Work out the finished part from the listing and answer in its coordinate system (mm). Face numbers are marked on the shaded views. Give positions to 0.01 mm unless a question says otherwise; leave off trailing zeros. Loops run counter-clockwise (first coordinate to the right, second up) from the corner with the lowest first, then second, coordinate; pieces in that order, holes last. Notation, with made-up numbers: (-17.75, 20) -> (32.25, 20) arc R24 cw to (32.25, 57) -> close; hole circle Ø9 at (-37, 57.5). An arc over 180 degrees is marked (long way). Answer as CSV lines item,"result". Start each with the question number.
1. Flat-ended cylindrical pins translate along their axes: pin 1 Ø2 at (x, y) = (-6, 1.5) entering from +Z; pin 2 Ø4 at (x, z) = (0, 0) entering from +Y; pin 3 Ø12 at (x, z) = (-5, -23) entering from +Y; pin 4 Ø4 at (x, y) = (-27.5, 5) entering from -Z. Find the tip coordinate at first contact, or state that the pin passes through.
2. Find section C-C, the plane y = 4. Give the vertices of the cut face in (x, z).
3. Find section D-D, the plane x = -6. Give the vertices of the cut face in (y, z), and give its area (3 significant figures).
4. Find the intervals of material crossed by line 1 along X through (y, z) = (6.5, -35); line 2 along Z through (x, y) = (-9.5, 8.75); line 3 along Z through (x, y) = (-14, 5.5), in increasing order.
5. Determine the mould class of the marked faces 1 and 2 for opening direction X: +X half, -X half, draft (parallel to the pull), parting line (faces both ways), or undercut.
6. Find section A-A, the plane x = 0. Give the vertices of the cut face in (y, z).
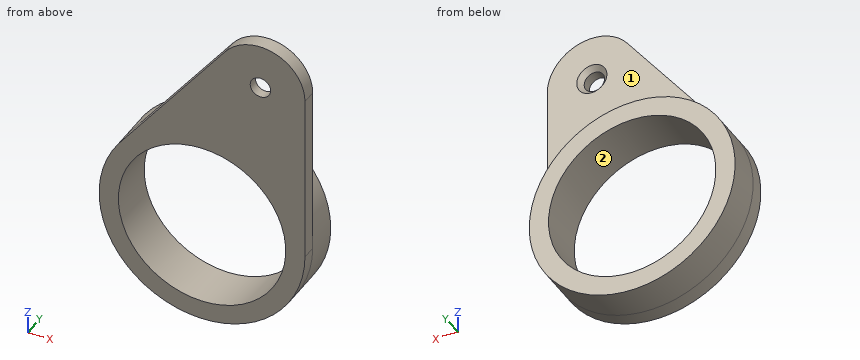
from build123d import *
from build123d.topology import SkipClean

# Parameters (mm, degrees)
SKETCH1_R           = 17.2
SKETCH1_R_2         = 2.1
BOSS_EXTRUDE1_DEPTH = 3
CHAMFER1_SIZE       = 1
SKETCH2_R           = 21.154971589
SKETCH2_R_2         = 17.2
BOSS_EXTRUDE2_DEPTH = 7


with BuildPart() as part:
    # Sketch1 → Boss-Extrude1 (new body)
    with BuildSketch(Plane(origin=(0, 0, 0), x_dir=(1, 0, 0), z_dir=(0, 1, 0))):
        with BuildLine():
            ThreePointArc((-29.22705293, 22.721503746), (-18.44573532, 55.149077376), (9.154971589, 35))
            Line((9.154971589, 35), (9.154971589, 0))
            ThreePointArc((9.154971589, 0), (2.966995431, -8.660856938), (-7.231849971, -5.613719871))
            Line((-7.231849971, -5.613719871), (-29.22705293, 22.721503746))
        make_face()
        with Locations(Location((-12, 35, 0), (0, 0, 270))):
            Circle(SKETCH1_R, mode=Mode.SUBTRACT)
        with Locations(Location((0, 0, 0), (0, 0, 270))):
            Circle(SKETCH1_R_2, mode=Mode.SUBTRACT)
    extrude(amount=BOSS_EXTRUDE1_DEPTH)

    # Chamfer1
    chamfer1_edges = [part.edges().sort_by_distance(p)[0] for p in [
        (0, 3, -2.1),
    ]]
    chamfer(chamfer1_edges, length=CHAMFER1_SIZE)

    # Sketch2 → Boss-Extrude2 (add)
    with SkipClean():  # the faces are left unmerged after this step: merging them gives an invalid solid
        with BuildSketch(Plane(origin=(0, 3, 0), x_dir=(1, 0, 0), z_dir=(0, 1, 0))):
            with Locations((-12, 35)):
                Circle(SKETCH2_R)
            with Locations(Location((-12, 35, 0), (0, 0, 270))):
                Circle(SKETCH2_R_2, mode=Mode.SUBTRACT)
        extrude(amount=BOSS_EXTRUDE2_DEPTH)


solid = part.part
Resolved:
1,pin 1,"stops at z = 7.67"
1,pin 2,"passes through"
1,pin 3,"stops at y = 10"
1,pin 4,"stops at z = -51.29"
2,outline,"circle Ø42.31 at (-12, -35); hole circle Ø34.4 at (-12, -35)"
3,outline,"(0, -55.29) -> (10, -55.29) -> (10, -51.12) -> (0, -51.12) -> close; (0, -18.88) -> (10, -18.88) -> (10, -14.71) -> (3, -14.71) -> (3, 6.91) -> (0, 6.91) -> close"
3,area,"148 mm^2"
4,line 1,"x = -33.15 to -29.2, 5.2 to 9.15"
4,line 2,"z = -56.01 to -52.02, -17.98 to -13.99"
4,line 3,"z = -56.06 to -52.08, -17.92 to -13.94"
5,face 1,"draft"
5,face 2,"undercut"
6,outline,"(0, -52.42) -> (10, -52.42) -> (10, -47.32) -> (0, -47.32) -> close; (0, -22.68) -> (10, -22.68) -> (10, -17.58) -> (3, -17.58) -> (3, -3.1) -> (2, -2.1) -> (0, -2.1) -> close; (0, 2.1) -> (2, 2.1) -> (3, 3.1) -> (3, 9.15) -> (0, 9.15) -> close"
